```python
from build123d import *

# Parameters (mm, degrees)
F1_DEPTH = 3
F2_R     = 1.5
F3_DEPTH = 2
F6_DEPTH = 25
F8_DEPTH = 25
F9_R     = 1.5


with BuildPart() as f1:
    # F0 (on Top) → F1 (new body)
    with BuildSketch(Plane.XY):
        Polygon((-9.8, 27), (-9.8, 0), (9.8, 0), (9.8, 27), (6.8, 27), (6.8, 12), (3.8, 12), (3.8, 27), (-3.8, 27), (-3.8, 12), (-6.8, 12), (-6.8, 27), align=None)
    extrude(amount=F1_DEPTH)

    # F2 (on face) → F3 (join)
    with BuildSketch(Plane.YZ.offset(9.8)):
        with Locations((25.5, 1.5)):
            Circle(F2_R)
    extrude(amount=F3_DEPTH)

    # F5: F1 across plane


with BuildPart() as f1_1:
    add(f1.part)
    add(f1.part.mirror(Plane(origin=(0, 12.8316278075, 1.5), x_dir=(0, 1, 0), z_dir=(1, 0, 0))))

    # F6 (cut): faces of the model
    f6_faces = [f1_1.faces().sort_by_distance(p)[0] for p in [
        (-9.8, 26.6649480916, 0.3350519084),
        (-9.8, 26.6649480916, 2.6649480916),
    ]]
    extrude(f6_faces, amount=-F6_DEPTH, mode=Mode.SUBTRACT)

    # F7 (on face) → F8 (cut)
    with BuildSketch(Plane.YZ.offset(9.8)):
        Polygon((0, 3), (0, 0), (2.5, 0), align=None)
    extrude(amount=-F8_DEPTH, mode=Mode.SUBTRACT)

    # F9
    f9_edges = [f1_1.edges().sort_by_distance(p)[0] for p in [
        (-9.8, 1.25, 1.5),
        (9.8, 1.25, 1.5),
    ]]
    fillet(f9_edges, radius=F9_R)


solid = f1_1.part
```
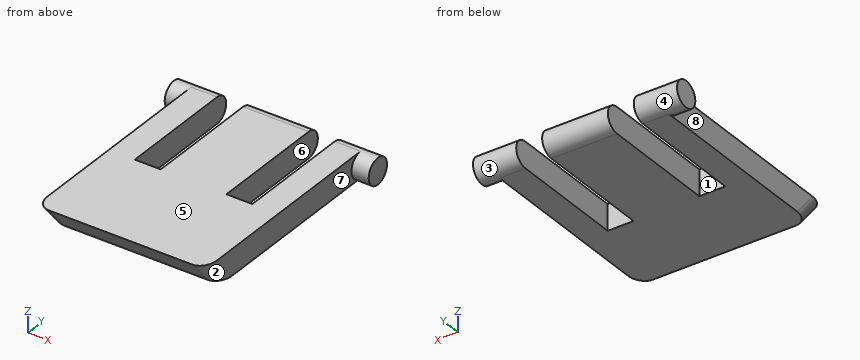
Design review of the part built by this model. Coordinates are the model's own, in mm. Face numbers are marked on the shaded views. A direction names the side the tool comes from. Coordinates: 2 decimals unless noted, no trailing zeros. Order: outer loops, then holes, each group sorted by start corner. A loop starts at its lowest first (then second) coordinate and runs counter-clockwise, first axis right, second up.
1) Mouldability with a two-part tool opening along X and no side actions: class the marked faces 6, 7 and 8 as +X half, -X half, draft (parallel to the pull), parting line (faces both ways), or undercut.
2) Take a section at A-A, the plane y = 16. Give the boundary of the cut face in (x, z), and give its area (3 significant figures).
3) Take a section at B-B, the plane x = -7.75. Give the boundary of the cut face in (y, z), and give its area (3 significant figures).
4) Clearance check with flat-ended pins moving along their axes: pin 1 (1 mm diameter, centred on x = -9.5, z = 0.5, fed in from +Y); pin 2 (0.9 mm diameter, centred on y = 21, z = 1, fed in from -X); pin 3 (1.5 mm diameter, centred on x = -5, z = 1.5, fed in from +Y). State where each tip first meets the part, or that it passes through.
5) Take a section at C-C, the plane x = 9.5. Give the boundary of the cut face in (y, z).
6) Wall thickness on line 1 along X through (y, z) = (21, 2.15); line 2 along X through (y, z) = (5.75, 0.7); line 3 along Y through (x, z) = (1.75, 2): over which ranges is each line inside the solid? List them lowest first.
7) For the marked faces 1, 2, 3, 4 and 5, list the 3-axis set-ups (+Z, -Z, +X, -X, +Y, -Y) from which the entire face can be reached by the end or side of a thin tool; tool diameter is ignored.
Returned:
1. face 6: undercut
1. face 7: +X half
1. face 8: -X half
2. outline: (-9.8, 0) - (-6.8, 0) - (-6.8, 3) - (-9.8, 3) - close; (-3.8, 0) - (3.8, 0) - (3.8, 3) - (-3.8, 3) - close; (6.8, 0) - (9.8, 0) - (9.8, 3) - (6.8, 3) - close
2. area: 40.8 mm2
3. outline: (0, 3) - (2.5, 0) - (25.5, 0) arc R1.5 ccw to (25.5, 3) - close
3. area: 76.3 mm2
4. pin 1: stops at y = 26.91
4. pin 2: stops at x = -9.8
4. pin 3: stops at y = 12
5. outline: (0.78, 3) - (3.28, 0) - (25.5, 0) arc R1.5 ccw to (25.5, 3) - close
6. line 1: x = -9.8 to -6.8, -3.8 to 3.8, 6.8 to 9.8
6. line 2: x = -9.8 to 9.8
6. line 3: y = 0.83 to 26.91
7. face 1: +Z, -Z, +Y
7. face 2: -Z, +X, -Y
7. face 3: +X
7. face 4: -X
7. face 5: +Z, +X, -X, +Y, -Y
